Design review of the part built by this model. Coordinates are the model's own, in mm. Coordinates: 2 decimals unless noted, no trailing zeros. Loops run counter-clockwise (first coordinate to the right, second up) from the corner with the lowest first, then second, coordinate; pieces in that order, holes last. Notation, with made-up numbers: M 23,-28.5 L 77,-28.5 A9 ccw 77,-24.5 Z; hole C 6,-12.75 d1. An arc over 180 degrees is marked long. One line per item, written item: value.
```python
from build123d import *

# Parameters (mm, degrees)
SKETCH_1_R      = 1.8
EXTRUDE_1_DEPTH = 18
FILLET_1_R      = 2


with BuildPart() as part:
    # 草图1 → 凸台-拉伸1 (new body)
    with BuildSketch(Plane(origin=(0, 0, 0), x_dir=(1, 0, 0), z_dir=(0, 1, 0))):
        with BuildLine():
            Line((0, -41.32), (0, -31.32))
            Line((0, -31.32), (0, -29.82))
            ThreePointArc((0, -29.82), (2.597888216, -29.706621767), (5.176021638, -29.367349216))
            ThreePointArc((5.176021638, -29.367349216), (5.775398606, -29.490339394), (6.277905634, -29.839432535))
            Line((6.277905634, -29.839432535), (8.333639143, -31.996940996))
            ThreePointArc((8.333639143, -31.996940996), (10.127846327, -33.082932859), (12.22492131, -33.111816408))
            ThreePointArc((12.22492131, -33.111816408), (12.877077837, -33.05487755), (13.512685008, -33.211573734))
            ThreePointArc((13.512685008, -33.211573734), (15.001951856, -34.459059049), (15.559656196, -36.32))
            Line((15.559656196, -36.32), (15.559656196, -41.32))
            Line((15.559656196, -41.32), (0, -41.32))
        make_face()
        with Locations(Location((5.176021638, -36.32, 0), (0, 0, 270))):
            Circle(SKETCH_1_R, mode=Mode.SUBTRACT)
        with Locations(Location((12.176021638, -36.32, 0), (0, 0, 270))):
            Circle(SKETCH_1_R, mode=Mode.SUBTRACT)
    extrude(amount=EXTRUDE_1_DEPTH)

    # 圆角1
    fillet_1_edges = [part.edges().sort_by_distance(p)[0] for p in [
        (15.559656196, 9, 41.32),
        (0, 9, 41.32),
    ]]
    fillet(fillet_1_edges, radius=FILLET_1_R)


solid = part.part
```
(1) Insertion check: pin 1 (2 mm diameter, centred on x = 12.5, y = 16, fed in from -Z). The pin has a flat end and moves straight along its axis. Give the tip position at first contact, or say it passes through.
Reply:
pin 1: stops at z = 33.05
(2) To check wall thickness, follow line 1 along X through (y, z) = (5.75, 36.32); line 2 along Z through (x, y) = (5.25, 14.75); line 3 along Z through (x, y) = (5.75, 15.25). State the ranges of each line that lie inside material, in increasing order. Write a range as [from, to].
Reply:
line 1: x = [0, 3.38], [6.98, 10.38], [13.98, 15.56]
line 2: z = [29.37, 34.52], [38.12, 41.32]
line 3: z = [29.48, 34.61], [38.03, 41.32]
(3) Mouldability with a two-part tool opening along X and no side actions: class faces 1 (the flat face through (7.29, 8.87, 30.9)), 2 (the flat face through (8, 9, 41.32)), 3 (the cylindrical face through (4.08, 8.87, 34.89)) as released by +X, released by -X, zero draft, split by the parting line, or undercut.
Reply:
face 1: released by +X
face 2: zero draft
face 3: undercut
(4) We need section A-A on x = 11. State the section outline as (y, z) points.
Reply:
outline: M 0,33.23 L 18,33.23 L 18,34.96 L 0,34.96 Z; M 0,37.68 L 18,37.68 L 18,41.32 L 0,41.32 Z
(5) We need section D-D on z = 32.5. State the section outline as (x, y) points.
Reply:
outline: M 0,0 L 8.92,0 L 8.92,18 L 0,18 Z
(6) We need section C-C on x = 3.75. State the section outline as (y, z) points, then the cut area to 3 significant figures.
Reply:
outline: M 0,29.58 L 18,29.58 L 18,35.22 L 0,35.22 Z; M 0,37.42 L 18,37.42 L 18,41.32 L 0,41.32 Z
area: 172 mm2
(7) We need section B-B on y = 4. State the section outline as (x, z) points.
Reply:
outline: M 0,29.82 A29.82 cw 5.18,29.37 A1.52 ccw 6.28,29.84 L 8.33,32 A4 cw 12.22,33.11 A2 ccw 13.51,33.21 A3.38 ccw 15.56,36.32 L 15.56,39.32 A2 ccw 13.56,41.32 L 2,41.32 A2 ccw 0,39.32 Z; hole C 5.18,36.32 d3.6; hole C 12.18,36.32 d3.6
